Autodesk Inventor part; units mm, degrees
sketch "Náčrt1" plane through (0, 0, 0) normal (0, 1, 0) x (-1, 0, 0)
  line L0 (0, 0) -> (-86, 0)
  line L1 (-86, 0) -> (-86, -55.5)
  line L2 (-86, -55.5) -> (0, -55.5)
  line L3 (0, -55.5) -> (0, 0)
  line L4 (0, -55.5) -> (0, -105.5)
  line L5 (0, -105.5) -> (-107, -105.5)
  line L6 (-107, -105.5) -> (-107, -55.5)
  line L7 (-107, -55.5) -> (-86, -55.5)
  dimension "d0" = 86
  dimension "d1" = 55.5
  dimension "d2" = 90
  dimension "d3" = 50
  dimension "d4" = 107
extrude "Vysunutí1" add sketch "Náčrt1" along normal blind 1.8
sketch "Náčrt2" plane through (0, 1.8, 0) normal (0, 1, 0) x (1, 0, 0)
  line L0 (107, 105.5) -> (0, 105.5)
  line L1 (107, 55.5) -> (107, 105.5)
  line L2 (86, 55.5) -> (107, 55.5)
  line L3 (86, 0) -> (86, 55.5)
  line L4 (0, 0) -> (86, 0)
  line L5 (0, 105.5) -> (0, 0)
  line L6 (85, 1) -> (85, 55.5)
  line L7 (14.5, 55.5) -> (14.5, 0)
  line L8 (15.5, 55.5) -> (85, 55.5)
  line L9 (1, 56.5) -> (106, 56.5)
  line L10 (1, 56.5) -> (1, 104.5)
  line L11 (1, 104.5) -> (106, 104.5)
  line L12 (106, 104.5) -> (106, 56.5)
  line L13 (15.5, 1) -> (85, 1)
  line L14 (15.5, 55.5) -> (15.5, 1)
  line L15 (14.5, 55.5) -> (1, 55.5)
  line L16 (1, 55.5) -> (1, 18)
  line L17 (1, 18) -> (14.5, 18)
  line L18 (0, 17) -> (14.5, 17)
  dimension "d21" = 14.5
  dimension "d22" = 1
  dimension "d23" = 1
  dimension "d24" = 48
  dimension "d25" = 105
  dimension "d28" = 1
  dimension "d29" = 37.5
  dimension "d30" = 1
  dimension "d31" = 1
  dimension "d45" = 1
  dimension "d46" = 1
  dimension "d47" = 1
  dimension "d48" = 54.5
  dimension "d49" = 1
  dimension "d50" = 1
  dimension "d51" = 69.5
extrude "Vysunutí3" add sketch "Náčrt2" along normal blind 4 contours L1 L2 L3 L4 L7 L18 L5 L0
sketch "Náčrt3" plane through (0, 1.8, 0) normal (0, 1, 0) x (1, 0, 0)
  line L0 (14.5, 17) -> (0, 17)
  line L1 (0, 17) -> (0, 0)
  line L2 (0, 0) -> (14.5, 0)
  line L3 (14.5, 0) -> (14.5, 17)
extrude "Vysunutí4" cut sketch "Náčrt3" against normal blind 4
sketch "Náčrt4" plane through (107, 0, -105.5) normal (0, 0, -1) x (-1, 0, 0)
  line L0 (101, 3.2) -> (94, 3.2)
  line L1 (101, 3.2) -> (101, 5.8)
  line L2 (101, 3.2) -> (103.6, 3.2) construction
  line L3 (94, 5.8) -> (94, 3.2)
  line L4 (0, 5.8) -> (107, 5.8)
  line L5 (107, 0) -> (107, 5.8)
  line L6 (106, 5.8) -> (92.5, 5.8)
  line L7 (101, 5.8) -> (92.5, 5.8)
  dimension "d37" = 7
  dimension "d39" = 90
  dimension "d41" = 6
  dimension "d42" = 3.6
sketch "Náčrt4 outline for Vysunutí5" plane through (107, 0, -105.5) normal (0, 0, -1) x (-1, 0, 0)
  line L0 (94, 3.2) -> (101, 3.2)
  line L1 (92.5, 5.8) -> (94, 3.2)
  line L2 (101, 5.8) -> (92.5, 5.8)
  line L3 (101, 3.2) -> (101, 5.8)
extrude "Vysunutí5" cut sketch "Náčrt4 outline for Vysunutí5" against normal blind 4
sketch "Sketch5" plane through (0, 0, 0) normal (0, 1, 0) x (-1, 0, 0)
  line L0 (-86, -55.5) -> (-107, -55.5)
  line L1 (-107, -55.5) -> (-107, -35.5)
  line L2 (-107, -35.5) -> (-86, -35.5)
  line L3 (-86, 0) -> (-86, -55.5)
  line L4 (0, -105.5) -> (0, -17)
  line L5 (0, -55.5) -> (12, -55.5)
  line L6 (12, -55.5) -> (12, -35.5)
  line L7 (12, -35.5) -> (0, -35.5)
  line L8 (0, -35.5) -> (0, -55.5)
  line L9 (-1, -55.5) -> (-14.5, -55.5)
  line L10 (0, -17) -> (-14.5, -17)
  point P0 (0, 0)
  dimension "d52" = 20
  dimension "d53" = 12
  dimension "d54" = 20
  dimension "d55" = 18.5
extrude "Extrusion6" add sketch "Sketch5" along normal blind 2
properties part number "Entrance_System"
Here's how the part is built. I have some questions about the finished solid (model axes, mm). A direction names the side the tool comes from. Round coordinates to 2 decimals unless told otherwise and drop trailing zeros. Loops run counter-clockwise (first coordinate to the right, second up) from the corner with the lowest first, then second, coordinate; pieces in that order, holes last. Notation, with made-up numbers: M 17.25,64.25 L 66.25,64.25 A33 cw 66.25,98.25 Z; hole C -37.5,24 d6. An arc over 180 degrees is marked long. Write each question's results on one line, items separated by ' | '. Start each with the question number.
(1) I want a section at D-D (z = -46.5). Please give me the cut outline in (x, y).
(2) Will these pins go through, and if not, where does the flat tip stop? P1, Ø10, axis at x = 35.5, z = -78.5, coming from the +Y side; P2, Ø1.2, axis at y = 4, z = -44.5, coming from the -X side; P3, Ø10, axis at x = 98.5, z = -48.5, coming from the +Y side.
(3) If I drill on probe 1 along X at (y, z) = (5.15, -20); probe 2 along Z at (x, y) = (58.5, 2.05); probe 3 along X at (y, z) = (4.95, -81.5), over which ranges is the centre line in solid material (lowest first)? Write a range as from..to.
(4) On a 3-axis mill with a long thin cutter (end or side, diameter ignored), from which of +Z, -Z, +X, -X, +Y, -Y can I reach the whole of each face in a straight line? I mean faces 1 (the flat face through (7, 3, -17)), 2 (the flat face through (8, 4, -55.5)), 3 (the flat face through (-6, 2, -45)), 4 (the flat face through (48, 0, -52)), 5 (the flat face through (97, 2, -45)). Say none if no direction works.
(5) I want a section at C-C (y = 4.1). Please give me the cut outline in (x, z), then the cut area to 3 significant figures.
(6) I want a section at A-A (z = -20). Please give me the cut outline in (x, y).
(7) I want a section at B-B (x = 71). Please give me the cut outline in (y, z), then the cut area to 3 significant figures.
Solved:
1) outline: M -12,0 L 107,0 L 107,2 L 86,2 L 86,5.8 L 85,5.8 L 85,1.8 L 15.5,1.8 L 15.5,5.8 L 14.5,5.8 L 14.5,1.8 L 1,1.8 L 1,5.8 L 0,5.8 L 0,2 L -12,2 Z
2) P1: stops at y = 1.8 | P2: stops at x = 0 | P3: stops at y = 2
3) probe 1: x = 0..1, 14.5..15.5, 85..86 | probe 2: z = -105.5..-104.5, -56.5..-55.5, -1..0 | probe 3: x = 0..1, 106..107
4) face 1: +Z, -X, +Y, -Y | face 2: +Y | face 3: +Z, -Z, -X, +Y | face 4: +Z, -Z, +X, -X, -Y | face 5: +Z, +X, +Y
5) outline: M 0,-105.5 L 6,-105.5 L 6,-104.5 L 1,-104.5 L 1,-56.5 L 106,-56.5 L 106,-104.5 L 13.52,-104.5 L 13.52,-105.5 L 107,-105.5 L 107,-55.5 L 86,-55.5 L 86,0 L 14.5,0 L 14.5,-17 L 0,-17 Z; hole M 1,-55.5 L 14.5,-55.5 L 14.5,-18 L 1,-18 Z; hole M 15.5,-55.5 L 85,-55.5 L 85,-1 L 15.5,-1 Z | area: 535 mm²
6) outline: M 0,0 L 86,0 L 86,5.8 L 85,5.8 L 85,1.8 L 15.5,1.8 L 15.5,5.8 L 14.5,5.8 L 14.5,1.8 L 1,1.8 L 1,5.8 L 0,5.8 Z
7) outline: M 0,-105.5 L 5.8,-105.5 L 5.8,-104.5 L 1.8,-104.5 L 1.8,-56.5 L 5.8,-56.5 L 5.8,-55.5 L 1.8,-55.5 L 1.8,-1 L 5.8,-1 L 5.8,0 L 0,0 Z | area: 202 mm²
